```python
from build123d import *

# Parameters (mm, degrees)
F0_R      = 20
F1_DEPTH  = 7.5
F2_R      = 17.5
F3_DEPTH  = 7.8
F4_R      = 20
F5_DEPTH  = 100
F6_R      = 25
F7_DEPTH  = 5
F8_SIZE   = 5
F9_R      = 15
F10_DEPTH = 115.3
F11_W     = 4
F11_H     = 15.3
F12_DEPTH = 25
F13_W     = 4
F13_H     = 15.3
F14_DEPTH = 25


with BuildPart() as f1:
    # F0 (on Top) → F1 (new body)
    with BuildSketch(Plane.XY):
        Circle(F0_R)
    extrude(amount=F1_DEPTH)

    # F2 (on face) → F3 (join)
    with BuildSketch(Plane.XY.offset(7.5)):
        Circle(F2_R)
    extrude(amount=F3_DEPTH)

    # F4 (on face) → F5 (join)
    with BuildSketch(Plane.XY.offset(15.3)):
        Circle(F4_R)
    extrude(amount=F5_DEPTH)

    # F6 (on face) → F7 (join)
    with BuildSketch(Plane.XY.offset(115.3)):
        Circle(F6_R)
    extrude(amount=F7_DEPTH)

    # F8
    f8_edges = [f1.edges().sort_by_distance(p)[0] for p in [
        (-20, 0, 0),
    ]]
    chamfer(f8_edges, length=F8_SIZE)

    # F9 (on face) → F10 (cut, through all)
    with BuildSketch(Plane(origin=(0, 0, 0), x_dir=(1, 0, 0), z_dir=(0, 0, -1))):
        Circle(F9_R)
    extrude(amount=-F10_DEPTH, mode=Mode.SUBTRACT)

    # F11 (on Front) → F12 (cut, symmetric)
    with BuildSketch(Plane.XZ):
        with Locations((0, 7.65)):
            Rectangle(F11_W, F11_H)
    extrude(amount=F12_DEPTH, both=True, mode=Mode.SUBTRACT)

    # F13 (on Right) → F14 (cut, symmetric)
    with BuildSketch(Plane.YZ):
        with Locations((0, 7.65)):
            Rectangle(F13_W, F13_H)
    extrude(amount=F14_DEPTH, both=True, mode=Mode.SUBTRACT)


solid = f1.part
```
Geometry check sheet. Reference: the model listing, model coordinates, mm. A direction names the side the tool comes from. Round coordinates to 2 decimals unless told otherwise and drop trailing zeros. Loops run counter-clockwise (first coordinate to the right, second up) from the corner with the lowest first, then second, coordinate; pieces in that order, holes last. Notation, with made-up numbers: M -10,-34 L 28,-34 A7 ccw 28,-29 Z; hole C 37.25,-25.5 d7. An arc over 180 degrees is marked long. Return JSON: item names as keys, results as strings. Group by question number.
(1) Go/stop test with flat-tipped pins: pin 1 (4 mm diameter, centred on y = -17.5, z = 6, fed in from -X); pin 2 (20 mm diameter, centred on x = -4.5, y = -6, fed in from -Z); pin 3 (6 mm diameter, centred on x = 15, z = 89.5, fed in from +Y); pin 4 (12 mm diameter, centred on y = 18.5, z = 46, fed in from -X). Record where each tip stops, or that it passes through.
(2) Mould release check, pull along X, two halves, no side actions. Record for faces 6 (the face through (-2, -16, 8)), 7 (the face through (-13, 12, 7.5)), 8 (the face through (-11.8, 12.1, 1.9)), 9 (the face through (23.846, 7.509, 117.765)): pulls with the +X half, pulls with the -X half, needs draft (parallel to the pull), parting line crosses it, or undercut.
(3) Set-up check for faces 1 (the face through (12, 13, 7.5)), 2 (the face through (2, -16, 8)), 3 (the face through (0, 16, 15.3)), 4 (the face through (16, -2, 8)), 5 (the face through (-14.006, 14.277, 6.232)): record each of +Z, -Z, +X, -X, +Y, -Y from which the full face is reachable in a straight line by a thin tool's end or side.
(4) Scan lines: line 1 along Y through (x, z) = (0, 32); line 2 along Z through (x, y) = (15, -18.5). Record each from-to range of solid material in increasing order. Write a range as [from, to].
(5) Section check D-D, the plane y = -21.5. Enter the section's corners in (x, z), and give its area (3 significant figures).
(6) Section check A-A, the plane x = 0. Enter the section's corners in (y, z).
(7) Section check C-C, the plane z = 33.5. Enter the section's corners in (x, y), and give its area (3 significant figures).
Data:
{
 "1": {"pin 1": "x = -12.64", "pin 2": "z = 0", "pin 3": "y = 16", "pin 4": "x = -15.61"},
 "2": {"face 6": "undercut", "face 7": "needs draft", "face 8": "pulls with the -X half", "face 9": "parting line crosses it"},
 "3": {"face 1": "+X, +Y", "face 2": "-Z, +Y, -Y", "face 3": "none", "face 4": "-Z, +X, -X", "face 5": "-Z, -X, +Y"},
 "4": {"line 1": "[-20, -15], [15, 20]", "line 2": "[115.3, 120.3]"},
 "5": {"outline": "M -12.76,115.3 L 12.76,115.3 L 12.76,120.3 L -12.76,120.3 Z", "area": "128 mm²"},
 "6": {"outline": "M -25,115.3 L -20,115.3 L -20,15.3 L -15,15.3 L -15,115.3 L 15,115.3 L 15,15.3 L 20,15.3 L 20,115.3 L 25,115.3 L 25,120.3 L -25,120.3 Z"},
 "7": {"outline": "C 0,0 d40; hole C 0,0 d30", "area": "550 mm²"}
}
